Job drawing, mm, ordinate dimensions from the low corner. One solid piece. A direction names the side the tool comes from. Give positions to 0.01 mm unless a question says otherwise; leave off trailing zeros. Order: outer loops, then holes, each group sorted by start corner. A loop starts at its lowest first (then second) coordinate and runs counter-clockwise, first axis right, second up.
1. Which spindle directions (+Z, -Z, +X, -X, +Y, -Y) get a long thin tool onto all of the face, cutting with end or side? Do the marked faces 5, 6 and 7. Say none if no direction does.
2. Drop flat-ended pins along their axis: pin 1 Ø5 at (x, y) = (12, 194.15) entering from -Z; pin 2 Ø1 at (x, y) = (51, 169) entering from -Z (1 decimal); pin 3 Ø16.5 at (x, z) = (34.5, 23.5) entering from -Y; pin 4 Ø20.5 at (x, z) = (37.5, 35) entering from +Y. Give the stop position or say it passes through.
3. Slice it at D-D on z = 31. List the corners of the cut face in (x, y), and give its area (3 significant figures).
4. Slice it at C-C on x = 12. List the corners of the cut face in (y, z), and give its area (3 significant figures).
5. Slice it at B-B on z = 13. List the corners of the cut face in (x, y), and give its area (3 significant figures).
6. Mould opens along X. For the marked faces 1, 2, 3 and 4 say: +X half, -X half, draft (parallel to the pull), parting line (faces both ways), or undercut.
7. Probe line 1 (Y direction, x = 68, z = 1.95); line 2 (Y direction, x = 54, z = 71); line 3 (X direction, y = 32, z = 71). List the from-to ranges inside material, lowest first.
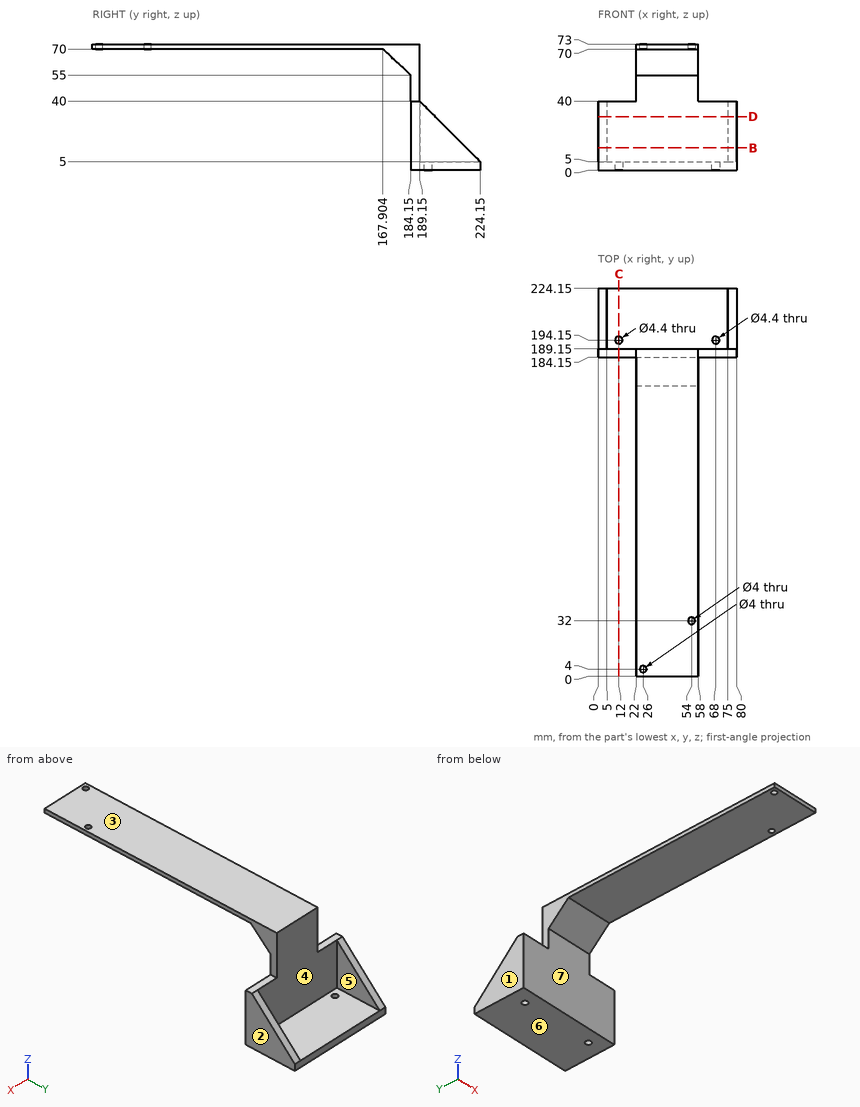
Data:
1. face 5: +Z, +Y
1. face 6: -Z, +X, -X, +Y, -Y
1. face 7: -Z, +X, -X, -Y
2. pin 1: stops at z = 0
2. pin 2: stops at z = 68.5
2. pin 3: stops at y = 184.15
2. pin 4: stops at y = 189.15
3. outline: (0, 184.15) - (80, 184.15) - (80, 198.15) - (75, 198.15) - (75, 189.15) - (5, 189.15) - (5, 198.15) - (0, 198.15) - close
3. area: 490 mm2
4. outline: (184.15, 0) - (191.95, 0) - (191.95, 5) - (189.15, 5) - (189.15, 40) - (184.15, 40) - close; (196.35, 0) - (224.15, 0) - (224.15, 5) - (196.35, 5) - close
4. area: 353 mm2
5. outline: (0, 184.15) - (80, 184.15) - (80, 216.15) - (75, 216.15) - (75, 189.15) - (5, 189.15) - (5, 216.15) - (0, 216.15) - close
5. area: 670 mm2
6. face 1: -X half
6. face 2: +X half
6. face 3: draft
6. face 4: undercut
7. line 1: y = 184.15 to 191.95, 196.35 to 224.15
7. line 2: y = 0 to 30, 34 to 189.15
7. line 3: x = 22 to 52, 56 to 58
